```python
from build123d import *

# Parameters (mm, degrees)
SKETCH1_R           = 4
BOSS_EXTRUDE1_DEPTH = 6.35
SKETCH1_3_R         = 10
SKETCH1_3_R_2       = 4
BOSS_EXTRUDE2_DEPTH = 20
BOSS_EXTRUDE3_START = -6
BOSS_EXTRUDE3_DEPTH = 6


with BuildPart() as part:
    # Sketch1 → Boss-Extrude1 (new body)
    with BuildSketch(Plane(origin=(0, 0, 0), x_dir=(1, 0, 0), z_dir=(0, 1, 0))):
        with BuildLine():
            Line((0, 0), (10.032558322, -30.806291758))
            ThreePointArc((10.032558322, -30.806291758), (20, -40), (29.967441678, -30.806291758))
            Line((29.967441678, -30.806291758), (40, 0))
            Line((40, 0), (0, 0))
        make_face()
        with Locations(Location((20, -30, 0), (0, 0, 270))):
            Circle(SKETCH1_R, mode=Mode.SUBTRACT)
    extrude(amount=BOSS_EXTRUDE1_DEPTH)

    # Sketch1_3 → Boss-Extrude2 (add)
    # profile 1 of 2: a face of its own
    with BuildSketch(Plane(origin=(0, 0, 0), x_dir=(1, 0, 0), z_dir=(0, 1, 0))):
        with Locations((20, -30)):
            Circle(SKETCH1_3_R)
        with Locations(Location((20, -30, 0), (0, 0, 270))):
            Circle(SKETCH1_3_R_2, mode=Mode.SUBTRACT)
    # profile 2 of 2: a face of its own
    with BuildSketch(Plane(origin=(0, 0, 0), x_dir=(1, 0, 0), z_dir=(0, 1, 0))):
        with BuildLine():
            Line((5.258465246, 0), (0, 0))
            Line((0, 0), (10.032558322, -30.806291758))
            ThreePointArc((10.032558322, -30.806291758), (10.577250525, -26.65159854), (12.776404659, -23.084823187))
            Line((12.776404659, -23.084823187), (5.258465246, 0))
        make_face()
    extrude(amount=BOSS_EXTRUDE2_DEPTH)

    # Sketch2 → Boss-Extrude3 (add)
    with BuildSketch(Plane(origin=(0, 20, 0), x_dir=(1, 0, 0), z_dir=(0, 1, 0)).offset(BOSS_EXTRUDE3_START)):
        with BuildLine():
            Line((40.034175669, 0), (0, 0))
            Line((0, 0), (10.032558322, -30.806291758))
            ThreePointArc((10.032558322, -30.806291758), (19.596525576, -20.008142896), (30, -30))
            ThreePointArc((30, -30), (29.991857104, -30.403474424), (29.967441678, -30.806291758))
            Line((29.967441678, -30.806291758), (40.034175669, 0))
        make_face()
    extrude(amount=BOSS_EXTRUDE3_DEPTH)


solid = part.part
```
CAD build for the part. Positions are in the model's coordinates, mm. Coordinates: 2 decimals unless noted, no trailing zeros. Write each loop counter-clockwise with the first axis right and the second up, starting at its lowest first coordinate (ties: lowest second). Pieces come first, ordered by that corner, then holes. Notation, with made-up numbers: (64.25, 34.25) -> (94.25, 34.25) arc R27 cw to (94.25, 63.25) -> close; hole circle Ø4 at (-37.75, 14). An arc over 180 degrees is marked (long way). Use CSV: the item, a comma, the result in double quotes. Start each with the question number.
Item 1: Two-plate mould, pull along Y, no slides. Class faces 1 (the flat face through (20, 0, 15)), 2 (the flat face through (9.07, 10.12, 11.7)), 3 (the flat face through (20, 5, 0)): +Y half, -Y half, draft (parallel to the pull), parting line (faces both ways), or undercut.
Item 2: Drop flat-ended pins along their axis: P1, Ø2, axis at y = 10, z = 18, coming from the -X side; P2, Ø8, axis at y = 2.5, z = 5, coming from the -X side; P3, Ø1, axis at y = 17.5, z = 5.5, coming from the +X side. Give the stop position or say it passes through.
Item 3: Band-saw the part on D-D, the plane z = 11. Write the cut outline in (x, y), plus the area to 3 significant figures.
Item 4: Wall check: probe 1 along Y at (x, z) = (29.5, 26); probe 2 along X at (y, z) = (6.25, 27); probe 3 along X at (y, z) = (12, 30). Give the ranges that are in metal, low to high.
Item 5: Band-saw the part on B-B, the plane z = 33. Write the cut outline in (x, y).
Item 6: Band-saw the part on A-A, the plane y = 3.25. Write the cut outline in (x, z), plus the area to 3 significant figures.
Response values:
1,face 1,"-Y half"
1,face 2,"undercut"
1,face 3,"draft"
2,P1,"stops at x = 5.54"
2,P2,"stops at x = 0.33"
2,P3,"stops at x = 38.4"
3,outline,"(3.58, 0) -> (36.42, 0) -> (36.42, 6.35) -> (8.84, 6.35) -> (8.84, 14) -> (36.44, 14) -> (36.44, 20) -> (3.58, 20) -> close"
3,area,"446 mm2"
4,probe 1,"y = 0 to 6.35, 14 to 20"
4,probe 2,"x = 8.79 to 17.35, 22.65 to 31.21"
4,probe 3,"x = 9.77 to 16, 24 to 30"
5,outline,"(10.46, 0) -> (17.35, 0) -> (17.35, 20) -> (10.46, 20) -> close; (22.65, 0) -> (29.54, 0) -> (29.54, 20) -> (22.65, 20) -> close"
6,outline,"(0, 0) -> (40, 0) -> (29.97, 30.81) arc R10 ccw to (10.03, 30.81) -> close; hole circle Ø8 at (20, 30)"
6,area,"1,010 mm2"
